Check sheet for the drawn part. Datum: minimum x, y, z corner. Units: mm. A direction names the side the tool comes from. Coordinates: 2 decimals unless noted, no trailing zeros. Loops run counter-clockwise (first coordinate to the right, second up) from the corner with the lowest first, then second, coordinate; pieces in that order, holes last. Notation, with made-up numbers: (52.5, 87) -> (96.5, 87) arc R18 ccw to (96.5, 118) -> close; hole circle Ø5 at (37, -33). An arc over 180 degrees is marked (long way). Use CSV: the item, a comma, the result in double quotes. Start each with the question number.
1. Gauge pin test, flat ends, axial feed: pin 1 (3 mm diameter, centred on y = 10, z = 54, fed in from -X); pin 2 (6 mm diameter, centred on x = 33, z = 12, fed in from +Y); pin 3 (8 mm diameter, centred on x = 29, y = 25.5, fed in from +Z); pin 4 (20.5 mm diameter, centred on x = 25.4, y = 25.4, fed in from +Z). Record the tip position at first contact, or that the pin passes through.
2. Release check for a two-part mould opening along X. For the marked faces 1, 2 and 3 record: pulls with the +X half, pulls with the -X half, needs draft (parallel to the pull), parting line crosses it, or undercut.
3. Sectioned sample at B-B, the plane z = 17. Record the cut outline in (x, y).
4. Set-up check for the marked faces 4 and 5: record each of +Z, -Z, +X, -X, +Y, -Y from which the full face is reachable in a straight line by a thin tool's end or side.
5. Sectioned sample at A-A, the plane z = 65. Record the cut outline in (x, y), and give its area (3 significant figures).
6. Thickness scan on L1, parallel to Y at x = 25, z = 32; L2, parallel to X at y = 26, z = 5; L3, parallel to Y at x = 25.4, z = 70.25. Record the ranges inside material, lowest first.
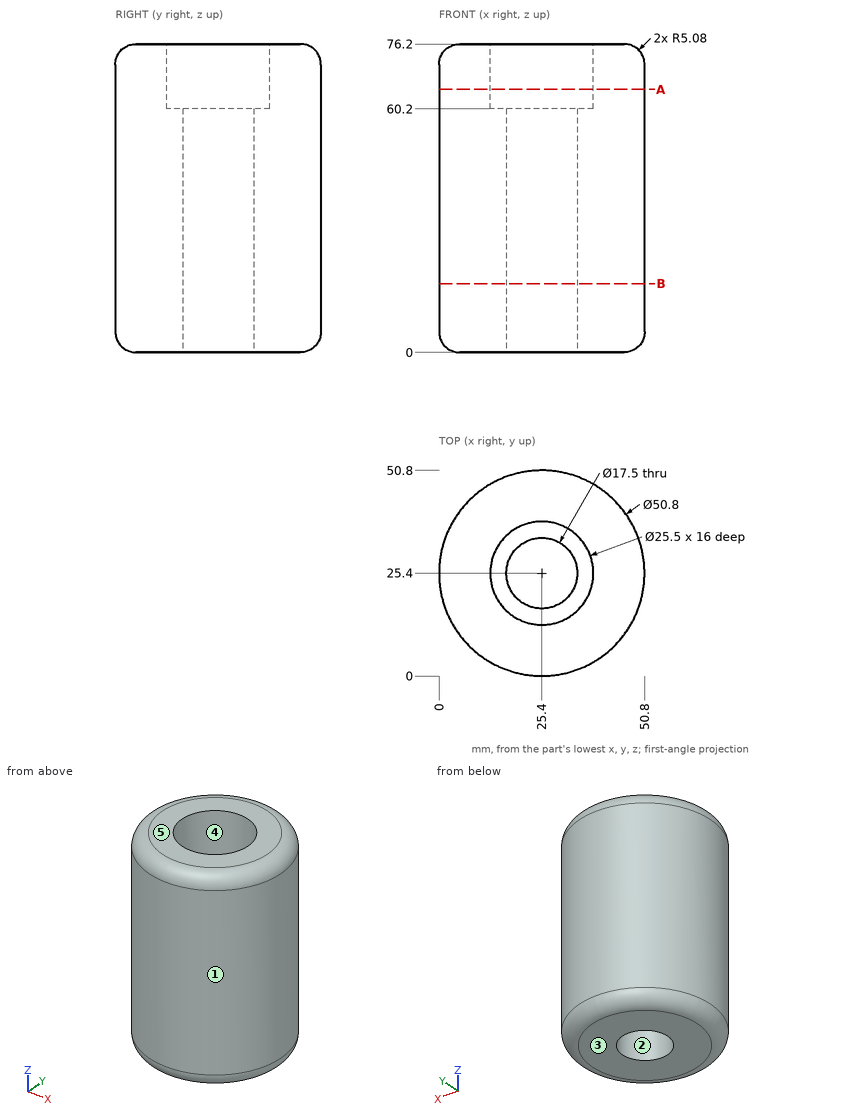
Completed:
1,pin 1,"x = 4.14"
1,pin 2,"y = 50.38"
1,pin 3,"through"
1,pin 4,"z = 60.2"
2,face 1,"parting line crosses it"
2,face 2,"undercut"
2,face 3,"needs draft"
3,outline,"circle Ø50.8 at (25.4, 25.4); hole circle Ø17.5 at (25.4, 25.4)"
4,face 4,"+Z"
4,face 5,"+Z, +X, -X, +Y, -Y"
5,outline,"circle Ø50.8 at (25.4, 25.4); hole circle Ø25.5 at (25.4, 25.4)"
5,area,"1,520 mm²"
6,L1,"0 to 16.66, 34.14 to 50.8"
6,L2,"0.01 to 16.67, 34.13 to 50.79"
6,L3,"0 to 12.65, 38.15 to 50.8"
